Verification items for the finished model (mm, model axes). A direction names the side the tool comes from. Give positions to 0.01 mm unless a question says otherwise; leave off trailing zeros. Loops run counter-clockwise (first coordinate to the right, second up) from the corner with the lowest first, then second, coordinate; pieces in that order, holes last. Notation, with made-up numbers: (30.5, 39.5) -> (77.5, 39.5) arc R22 cw to (77.5, 75.5) -> close; hole circle Ø2 at (-24.5, 86.25). An arc over 180 degrees is marked (long way). Use one line per item in the form item = value. Start each with the question number.
from build123d import *

# Parameters (mm, degrees)
F0_R     = 7.9
F0_R_2   = 6.35
F1_DEPTH = 15.875
F0_R_3   = 2.38125
F2_DEPTH = 31.75
F0_R_4   = 16.1925
F0_R_5   = 1.905
F4_DEPTH = 3.175
F6_DEPTH = 2.2


with BuildPart() as f1:
    # F0 (on Top) → F1 (new body)
    with BuildSketch(Plane.XY):
        Circle(F0_R)
        Circle(F0_R_2, mode=Mode.SUBTRACT)
    extrude(amount=F1_DEPTH)

    # F0 (on Top) → F2 (join)
    with BuildSketch(Plane.XY):
        Circle(F0_R_2)
        Circle(F0_R_3, mode=Mode.SUBTRACT)
    extrude(amount=F2_DEPTH)

    # F0 (on Top) → F4 (join)
    with BuildSketch(Plane.XY):
        Circle(F0_R_4)
        with Locations((0, -11.7475)):
            Circle(F0_R_5, mode=Mode.SUBTRACT)
        with Locations((-11.7475, 0)):
            Circle(F0_R_5, mode=Mode.SUBTRACT)
        Circle(F0_R, mode=Mode.SUBTRACT)
        with Locations((11.7475, 0)):
            Circle(F0_R_5, mode=Mode.SUBTRACT)
        with Locations((0, 11.7475)):
            Circle(F0_R_5, mode=Mode.SUBTRACT)
    extrude(amount=F4_DEPTH)

    # F5 (on face) → F6 (cut)
    with BuildSketch(Plane.XY.offset(31.75)):
        with BuildLine():
            ThreePointArc((6.35, 0), (6.3259541524, 0.5520906279), (6.2539987208, 1.1))
            Line((6.2539987208, 1.1), (2.1119544414, 1.1))
            ThreePointArc((2.1119544414, 1.1), (2.3129465057, 0.5662420193), (2.38125, 0))
            ThreePointArc((2.38125, 0), (2.3129465057, -0.5662420193), (2.1119544414, -1.1))
            Line((2.1119544414, -1.1), (6.2539987208, -1.1))
            ThreePointArc((6.2539987208, -1.1), (6.3259541524, -0.5520906279), (6.35, 0))
        make_face()
        with BuildLine():
            Line((-2.1119544414, 1.1), (-6.2539987208, 1.1))
            ThreePointArc((-6.2539987208, 1.1), (-6.35, 0), (-6.2539987208, -1.1))
            Line((-6.2539987208, -1.1), (-2.1119544414, -1.1))
            ThreePointArc((-2.1119544414, -1.1), (-2.38125, 0), (-2.1119544414, 1.1))
        make_face()
    extrude(amount=-F6_DEPTH, mode=Mode.SUBTRACT)


solid = f1.part
Item 1: Material ranges on line 1 (Y direction, x = 0, z = 1); line 2 (Z direction, x = 9, y = -5) (3 decimals); line 3 (X direction, y = -11, z = 2), recorded low to high.
Item 2: Gauge pin test, flat ends, axial feed: pin 1 Ø1.8 at (x, z) = (-4, 31) entering from -Y; pin 2 Ø10 at (x, y) = (-6, 12) entering from +Z (3 decimals); pin 3 Ø8 at (x, y) = (-5.5, -5.5) entering from -Z; pin 4 Ø2.5 at (x, z) = (5, 31) entering from -Y. Record the tip position at first contact, or that the pin passes through.
Item 3: Sectioned sample at D-D, the plane x = -13. Enter the section's corners in (y, z) (3 decimals), and give its area (3 significant figures).
Item 4: Tool access check on faces 5 (the cylindrical face through (-6.269, -4.807, 9.436)), 6 (the flat face through (0, -4, 31.75)), 7 (the flat face through (4, -1.1, 31)). Record the directions out of +Z, -Z, +X, -X, +Y, -Y that give a thin tool (end or side, any length) a straight path to the whole face; none if there is none.
Item 5: Sectioned sample at C-C, the plane z = 12. Enter the section's corners in (x, y).
Item 6: Draft check along X on faces 1 (the cylindrical face through (6.057, 1.907, 23.701)), 2 (the cylindrical face through (-0.413, 9.888, 1.565)), 3 (the cylindrical face through (-0.413, -13.607, 1.565)), 4 (the flat face through (-4, 1.1, 31)). Enter one of: +X half, -X half, draft (parallel to the pull), parting line (faces both ways), or undercut.
Item 7: Sectioned sample at A-A, the plane y = 0. State how many separate pieces and enclosed holes the cut face has, and give its area (3 significant figures).
Outcome:
q1.line_1 = -16.19 to -13.65, -9.84 to -2.38, 2.38 to 9.84, 13.65 to 16.19
q1.line_2 = 0 to 3.175
q1.line_3 = -11.88 to -1.75, 1.75 to 11.88
q2.pin_1 = -5.54
q2.pin_2 = 3.175
q2.pin_3 = 0
q2.pin_4 = -5.12
q3.outline = (-9.654, 0) -> (-1.435, 0) -> (-1.435, 3.175) -> (-9.654, 3.175) -> close; (1.435, 0) -> (9.654, 0) -> (9.654, 3.175) -> (1.435, 3.175) -> close
q3.area = 52.2 mm^2
q4.face_5 = +Z
q4.face_6 = +Z, +X, -X, +Y, -Y
q4.face_7 = +Z, +X, -X
q5.outline = circle Ø15.8 at (0, 0); hole circle Ø4.76 at (0, 0)
q6.face_1 = parting line
q6.face_2 = undercut
q6.face_3 = undercut
q6.face_4 = draft
q7.separate_pieces = 4
q7.enclosed_holes = 0
q7.area = 312 mm^2
